Model file for the job. Use its own axes, mm. A direction names the side the tool comes from. Round coordinates to 2 decimals unless told otherwise and drop trailing zeros. Loops run counter-clockwise (first coordinate to the right, second up) from the corner with the lowest first, then second, coordinate; pieces in that order, holes last. Notation, with made-up numbers: M 81.5,26.5 L 117.5,26.5 A9 cw 117.5,33.5 Z; hole C 88.25,59.25 d5. An arc over 180 degrees is marked long. Use a Markdown table: item, result. Add a question column.
Q1. Tool access for faces 1 (the face through (-50.344, 13.691, 9.86)), 2 (the face through (-45.18, 12.74, 9.86)): list every direction of +Z, -Z, +X, -X, +Y, -Y with a clear straight run to the whole face (end or side of a thin tool).
Q2. Probe line 1 (Z direction, x = -10, y = 1.3); line 2 (Y direction, x = -43, z = 10.25); line 3 (Y direction, x = -45.5, z = 15.5). List the from-to ranges inside material, lowest first. Write a range as from..to.
Q3. Cut at D-D (y = 15.75). Give the cut face in (x, z).
Q4. Mould opens along Z. For faces 3 (the face through (-31.7, 4.7, 0)), 4 (the face through (-31.7, 4.7, 20)), 5 (the face through (-30.54, 2.46, 7.56)) say: +Z half, -Z half, draft (parallel to the pull), parting line (faces both ways), or undercut.
Q5. Pin check, flat tips, straight feed: pin 1 (4 mm diameter, centred on x = -30, z = 10, fed in from +Y); pin 2 (12 mm diameter, centred on x = -10.5, z = 16.5, fed in from -Y); pin 3 (10 mm diameter, centred on y = 19, z = 14.5, fed in from -X); pin 4 (10 mm diameter, centred on y = 12.5, z = 9, fed in from -X). Stop position of each tip, or through.
Q6. Cut at B-B (z = 10). Give the cut face in (x, y), plus the area to 3 significant figures.
Q7. Cut at C-C (z = 1.25). Give the cut face in (x, y), plus the area to 3 significant figures.
Q8. Cut at A-A (x = -11.5). Give the cut face in (y, z), plus the area to 3 significant figures.
Autodesk Inventor part; units mm, degrees
ref_plane "YZ Plane" through (0, 0, 0) normal (1, 0, 0) x (0, 1, 0)
ref_plane "XZ Plane" through (0, 0, 0) normal (0, 1, 0) x (-1, 0, 0)
ref_plane "XY Plane" through (0, 0, 0) normal (0, 0, 1) x (1, 0, 0)
sketch "スケッチ1" plane through (0, 0, 0) normal (0, 0, 1) x (1, 0, 0)
  line L0 (0, 0) -> (-55, 0)
  line L1 (-55, 0) -> (-55, 5)
  line L2 (-55, 5) -> (-45.5551, 22.6294)
  line L3 (-45.5551, 22.6294) -> (-41.1478, 20.2682)
  line L4 (-41.1478, 20.2682) -> (-49.3276, 5)
  line L5 (-49.3276, 5) -> (0, 5)
  line L6 (0, 5) -> (0, 0)
  dimension "d0" = 61.82
  dimension "d1" = 55
  dimension "d2" = 5
  dimension "d3" = 5
  dimension "d4" = 20
extrude "押し出し1" add sketch "スケッチ1" along normal blind 20
sketch "スケッチ2" plane through (-55, 0, 0) normal (0, -1, 0) x (1, 0, 0)
  line L0 (55, 0) -> (55, 20)
  line L1 (55, 10) -> (45, 10) construction
  circle A0 centre (45, 10) radius 2.5
  circle A1 centre (25, 10) radius 2.5
  dimension "d7" = 5
  dimension "d8" = 10
  dimension "d11" = 20
extrude "押し出し2" cut sketch "スケッチ2" against normal up to next
properties part number "防水5_3D プリント"
Checked values:
| question | item | result |
|---|---|---|
| 1 | face 1 | +Z, -Z, -X, +Y |
| 1 | face 2 | +Z, -Z, +X |
| 2 | line 1 | z = 0..7.5, 12.5..20 |
| 2 | line 2 | y = 0..5, 16.81..21.26 |
| 2 | line 3 | y = 0..5, 12.14..22.6 |
| 3 | outline | M -49.24,0 L -43.57,0 L -43.57,20 L -49.24,20 Z |
| 4 | face 3 | -Z half |
| 4 | face 4 | +Z half |
| 4 | face 5 | undercut |
| 5 | pin 1 | passes through |
| 5 | pin 2 | stops at y = 0 |
| 5 | pin 3 | stops at x = -50.18 |
| 5 | pin 4 | stops at x = -53.66 |
| 6 | outline | M -55,0 L -32.5,0 L -32.5,5 L -49.33,5 L -41.15,20.27 L -45.56,22.63 L -55,5 Z; M -27.5,0 L -12.5,0 L -12.5,5 L -27.5,5 Z; M -7.5,0 L 0,0 L 0,5 L -7.5,5 Z |
| 6 | area | 318 mm^2 |
| 7 | outline | M -55,0 L 0,0 L 0,5 L -49.33,5 L -41.15,20.27 L -45.56,22.63 L -55,5 Z |
| 7 | area | 368 mm^2 |
| 8 | outline | M 0,0 L 5,0 L 5,8 L 0,8 Z; M 0,12 L 5,12 L 5,20 L 0,20 Z |
| 8 | area | 80.0 mm^2 |
